Autodesk Inventor part; units mm, degrees
ref_plane "YZ Plane" through (0, 0, 0) normal (1, 0, 0) x (0, 1, 0)
ref_plane "XZ Plane" through (0, 0, 0) normal (0, 1, 0) x (-1, 0, 0)
ref_plane "XY Plane" through (0, 0, 0) normal (0, 0, 1) x (1, 0, 0)
sketch "Sketch1" plane through (0, 0, 0) normal (0, 0, 1) x (1, 0, 0)
  circle A0 centre (0, 0) radius 3.5
  line L0 (0, 0) -> (7.5, 0)
  line L1 (0, 0) -> (-7.5, 0)
  line L2 (7.5, 0) -> (7.5, -18.1083)
  line L3 (-7.5, 0) -> (-7.5, -18.1083)
  circle A1 centre (7.5, -18.1083) radius 2.25
  circle A2 centre (-7.5, -18.1083) radius 2.25
  circle A3 centre (0, 0) radius 22.5
  line L4 (0, 0) -> (20.25, 0)
  line L5 (20.25, 0) -> (20.25, 9.8075)
  line L6 (0, 0) -> (-20.25, 0)
  line L7 (-20.25, 0) -> (-20.25, 9.8075)
  circle A4 centre (20.25, 9.8075) radius 2.25
  circle A5 centre (-20.25, 9.8075) radius 2.25
  line L8 (-20.25, 9.8075) -> (20.25, 9.8075)
  line L9 (20.25, 9.8075) -> (7.5, -18.1083)
  line L10 (7.5, -18.1083) -> (-7.5, -18.1083)
  line L11 (-7.5, -18.1083) -> (-20.25, 9.8075)
  line L12 (-20.25, 15.8075) -> (20.25, 15.8075)
  line L13 (25.7077, 7.3148) -> (12.9577, -20.601)
  line L14 (7.5, -24.1083) -> (-7.5, -24.1083)
  line L15 (-12.9577, -20.601) -> (-25.7077, 7.3148)
  circle A6 centre (-20.25, 9.8075) radius 6
  circle A7 centre (20.25, 9.8075) radius 6
  circle A8 centre (7.5, -18.1083) radius 6
  arc A9 (-13.499, -18.0007) -> (-7.5, -24.1083) centre (-7.5, -18.1083) ccw
  arc A10 (-7.5, -18.1083) -> (7.5, -18.1083) centre (0, 0) ccw
  dimension "d0" = 7
  dimension "d1" = 7.5
  dimension "d2" = 7.5
  dimension "d4" = 4.5
  dimension "d5" = 4.5
  dimension "d6" = 45
  dimension "d7" = 20.25
  dimension "d8" = 20.25
  dimension "d9" = 4.5
  dimension "d10" = 4.5
  dimension "d11" = 6
  dimension "d27" = 12
  dimension "d28" = 6
  dimension "d29" = 12
  dimension "d30" = 12
extrude "Extrusion1" add sketch "Sketch1" along normal blind 6 contours L0 L2 A8 L10 A2 L3 L1 A0 | A0 L1 L6 L11 A6 L8 A7 L9 L4 L0 | L4 L9 A8 L2 | L3 A2 L11 L6 | A8 L9 A1 L2 | L2 A1 L10 A8 | L9 A7 L5 L4 | L4 L5 A7 A3 L13 A8 L9 | L11 A2 A10 A8 A3 L15 A6 L7 L6 | L6 L7 A6 L11 | A8 A3 A10 A1 L9 | A8 A10 A2 L10 | L10 A1 A10 A8 | A7 L8 A4 L9 | L9 A4 L5 A7 | A6 L7 A5 L11 | L11 A5 L8 A6 | A8 A3 | A3 L13 A8 | L5 A4 A3 A7 | A7 A3 A4 L8 | L8 A6 A3 L12 A7 | A6 A3 A5 L7 | L8 A5 A3 A6 | A8 L14 A9 A3 | A7 L13 A3 | A3 A4 A7 | A3 L12 A7 | A6 A3 A5 | A3 L15 A6 | A6 L12 A3 | A9 L15 A3
sketch "Sketch2" plane through (0, 0, 0) normal (0, 0, -1) x (-1, 0, 0)
  circle A0 centre (0, 0) radius 3.5
  circle A1 centre (0, 0) radius 6.5
  circle A2 centre (0, 0) radius 3.5
  dimension "d14" = 13
extrude "Extrusion2" add sketch "Sketch2" along normal blind 4.5
fillet "Fillet1" radius 3 1 edges at (6.5, 0, 0)
sketch "Sketch3" plane through (0, 0, 6) normal (0, 0, 1) x (1, 0, 0)
  circle A0 centre (-20.25, 9.8075) radius 2.25
  arc A1 (-20.25, 15.8075) -> (-25.7077, 7.3148) centre (-20.25, 9.8075) ccw
  circle A2 centre (-20.25, 9.8075) radius 4.125
  circle A3 centre (-20.25, 9.8075) radius 2.25
  dimension "d18" = 8.25
  dimension "d36" = 4.5
extrude "Extrusion3" add sketch "Sketch3" along normal blind 4.5
sketch "Sketch4" plane through (-20.25, 9.8075, 10.5) normal (0, 0, 1) x (1, 0, 0)
  circle A0 centre (0, 0) radius 2.25
  circle A1 centre (0, 0) radius 4.125
  circle A2 centre (0, 0) radius 3.5
  circle A3 centre (0, 0) radius 2.25
  point P0 (20.25, -9.8075)
  dimension "d21" = 7
extrude "Extrusion4" add sketch "Sketch4" along normal blind 1.5 contours A2
sketch "Sketch5" plane through (-20.25, 9.8075, 12) normal (0, 0, 1) x (1, 0, 0)
  circle A0 centre (0, 0) radius 2.25
  circle A1 centre (0, 0) radius 3.5
  circle A2 centre (0, 0) radius 4.125
  circle A3 centre (0, 0) radius 2.25
  point P0 (20.25, -9.8075)
  dimension "d24" = 8.25
extrude "Extrusion5" add sketch "Sketch5" along normal blind 2.5 contours A1 | A2
sketch "Sketch6" plane through (0, 0, 6) normal (0, 0, 1) x (1, 0, 0)
  circle A0 centre (0, 0) radius 3.5
  line L0 (6.6973, 0) -> (3.3486, -5.8)
  line L1 (3.3486, -5.8) -> (-3.3486, -5.8)
  line L2 (-3.3486, -5.8) -> (-6.6973, 0)
  line L3 (-6.6973, 0) -> (-3.3486, 5.8)
  line L4 (-3.3486, 5.8) -> (3.3486, 5.8)
  line L5 (3.3486, 5.8) -> (6.6973, 0)
  circle A1 centre (0, 0) radius 9
  dimension "d31" = 11.6
  dimension "d32" = 18
extrude "Extrusion6" add sketch "Sketch6" along normal blind 4 contours A1
fillet "Fillet2" radius 2 1 edges at (-9, 0, 6)
draft "FaceDraft1" angle 22 pull direction (0, 0, 1) faces at (-16.1384, 9.4756, 9) fixed edges at (-24.375, 9.8075, 10.5)
properties part number "hexagon_1"
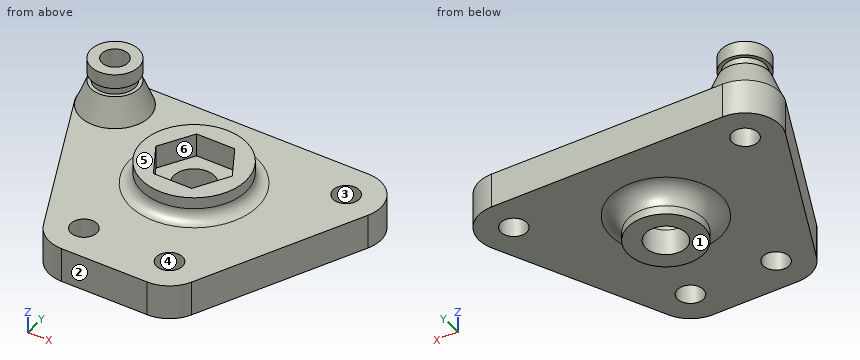
The listing builds one solid part. Answer for the finished solid, in the listing's coordinates (mm). Face numbers are marked on the shaded views. A direction names the side the tool comes from. Give positions to 0.01 mm unless a question says otherwise; leave off trailing zeros. Write each loop counter-clockwise with the first axis right and the second up, starting at its lowest first coordinate (ties: lowest second). Pieces come first, ordered by that corner, then holes. Notation, with made-up numbers: (1.25, 21.5) - (41.25, 21.5) arc R33 ccw to (41.25, 49.5) - close; hole circle Ø8 at (83, 26). An arc over 180 degrees is marked (long way). Use one line per item in the form item = value. Start each with the question number.
1) Find section C-C on z = 4.5. Determine the outline of the cut face in (x, y), plus the area to 3 significant figures.
2) Consider line 1 along Y through (x, z) = (-7.5, 1.4); line 2 along Y through (x, z) = (0, 1.7); line 3 along Z through (x, y) = (-7, -21.5). Determine where each line is inside the solid, lowest interval first. Write a range as from..to.
3) A tool of negligible diameter and unlimited length cuts with its end or side. For the marked faces 4, 5 and 6, from which of +Z, -Z, +X, -X, +Y, -Y can it reach the whole face along a straight path? Write none if from no direction.
4) Find section B-B on z = 9.25. Determine the outline of the cut face in (x, y).
5) Find section D-D on x = 21.5. Determine the outline of the cut face in (y, z).
6) Flat-ended cylindrical pins translate along their axes: pin 1 Ø6 at (y, z) = (2, 0.5) entering from +X; pin 2 Ø4 at (x, z) = (-9, 3.5) entering from -Y; pin 3 Ø20 at (x, y) = (12, -7) entering from +Z; pin 4 Ø1.5 at (x, y) = (9, -5) entering from +Z. Find the tip coordinate at first contact, or state that the pin passes through.
7) The mould has two halves that part along Y. Classify the marked faces 1, 2 and 3: pulls with the +Y half, pulls with the -Y half, needs draft (parallel to the pull), parting line crosses it, or undercut.
8) Find section A-A on x = 0. Determine the outline of the cut face in (y, z).
Geometry results:
q1.outline = (-25.71, 7.31) - (-12.96, -20.6) arc R6 ccw to (-7.5, -24.11) - (7.5, -24.11) arc R6 ccw to (12.96, -20.6) - (25.71, 7.31) arc R6 ccw to (20.25, 15.81) - (-20.25, 15.81) arc R6 ccw to start; hole circle Ø4.5 at (-20.25, 9.81); hole circle Ø4.5 at (-7.5, -18.11); hole circle Ø7 at (0, 0); hole circle Ø4.5 at (7.5, -18.11); hole circle Ø4.5 at (20.25, 9.81)
q1.area = 1,490 mm2
q2.line_1 = -24.11..-20.36, -15.86..15.81
q2.line_2 = -24.11..-3.5, 3.5..15.81
q2.line_3 = 0..6
q3.face_4 = +Z, -Z
q3.face_5 = +Z, +X, +Y, -Y
q3.face_6 = +Z
q4.outline = circle Ø9.26 at (-20.25, 9.81); circle Ø18 at (0, 0); hole circle Ø4.5 at (-20.25, 9.81); hole (-6.7, 0) - (-3.35, -5.8) - (3.35, -5.8) - (6.7, 0) - (3.35, 5.8) - (-3.35, 5.8) - close
q5.outline = (-1.9, 0) - (7.94, 0) - (7.94, 6) - (-1.9, 6) - close; (11.68, 0) - (15.68, 0) - (15.68, 6) - (11.68, 6) - close
q6.pin_1 = 24.65
q6.pin_2 = -24.11
q6.pin_3 = 10
q6.pin_4 = 6.63
q7.face_1 = needs draft
q7.face_2 = pulls with the -Y half
q7.face_3 = undercut
q8.outline = (-24.11, 0) - (-9.5, 0) arc R3 cw to (-6.5, -3) - (-6.5, -4.5) - (-3.5, -4.5) - (-3.5, 6) - (-5.8, 6) - (-5.8, 10) - (-9, 10) - (-9, 8) arc R2 cw to (-11, 6) - (-24.11, 6) - close; (3.5, -4.5) - (6.5, -4.5) - (6.5, -3) arc R3 cw to (9.5, 0) - (15.81, 0) - (15.81, 6) - (11, 6) arc R2 cw to (9, 8) - (9, 10) - (5.8, 10) - (5.8, 6) - (3.5, 6) - close
